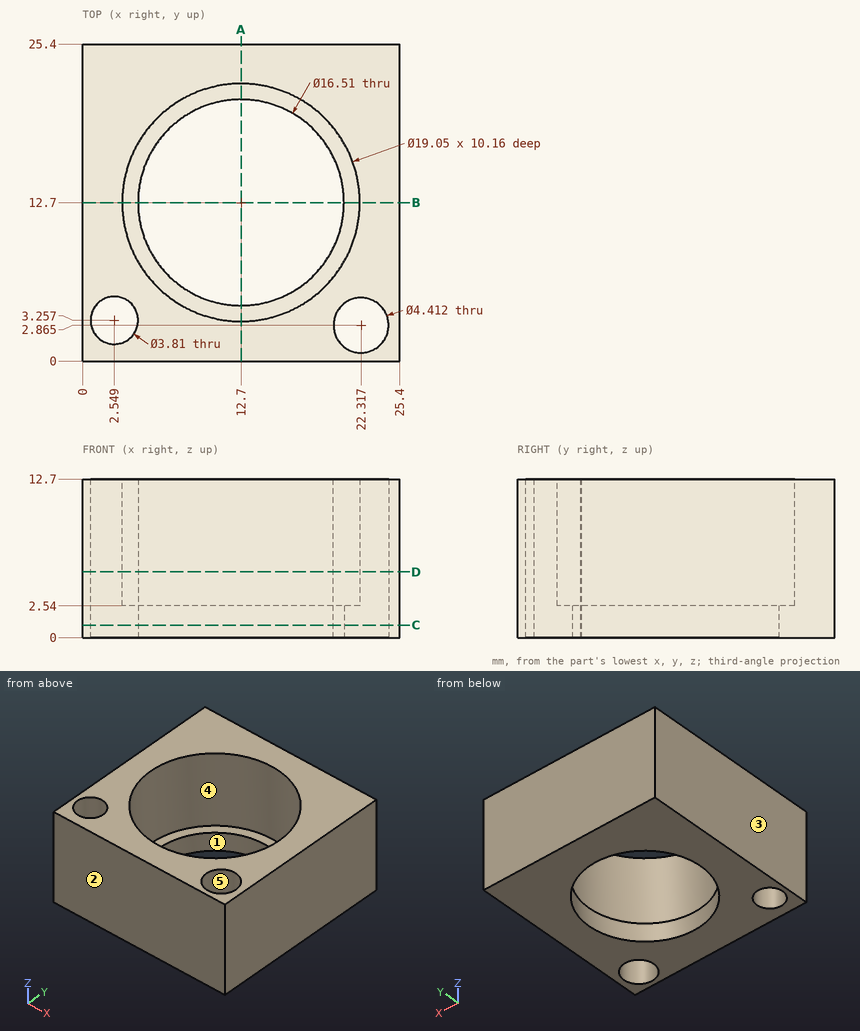
Here's the drawing with two shaded views (mm, measured from the low corner). I have some questions. A direction names the side the tool comes from. Give positions to 0.01 mm unless a question says otherwise; leave off trailing zeros. Order: outer loops, then holes, each group sorted by start corner. A loop starts at its lowest first (then second) coordinate and runs counter-clockwise, first axis right, second up. Notation, with made-up numbers: M 34,-3.5 L 89,-3.5 A5 cw 89,0.5 Z; hole C 2,37.5 d6. An arc over 180 degrees is marked long. Answer as a JSON object with one key per item and string values. Group by question number.
1) On a 3-axis mill with a long thin cutter (end or side, diameter ignored), from which of +Z, -Z, +X, -X, +Y, -Y can I reach the whole of each face in a straight line? I mean the marked faces 4 and 5. Say none if no direction works.
2) Suppose I cut it at C-C, the plane z = 1. Write out the boundary of the cut face in (x, y) (1 decimal).
3) Please list where these lines run through material, in increasing order: L1, parallel to Y at x = 12.7, z = 1.35 (1 decimal); L2, parallel to X at y = 3, z = 10.5 (1 decimal); L3, parallel to Y at x = 13, z = 9.5. Write a range as [from, to].
4) We'd pull the mould along X, two halves only. Please class the marked faces 1, 2 and 3: pulls with the +X half, pulls with the -X half, needs draft (parallel to the pull), parting line crosses it, or undercut.
5) Suppose I cut it at D-D, the plane z = 5.25. Count the separate pieces of the cut face and the enclosed holes in it.
6) Suppose I cut it at A-A, the plane x = 12.7. Write out the boundary of the cut face in (y, z) (1 decimal), plus the area to 3 significant figures.
Results found:
{
 "1": {"face 4": "+Z", "face 5": "+Z, -Z"},
 "2": {"outline": "M 0,0 L 25.4,0 L 25.4,25.4 L 0,25.4 Z; hole C 2.5,3.3 d3.8; hole C 12.7,12.7 d16.5; hole C 22.3,2.9 d4.4"},
 "3": {"L1": "[0, 4.4], [21, 25.4]", "L2": "[0, 0.7], [4.4, 20.1], [24.5, 25.4]", "L3": "[0, 3.18], [22.22, 25.4]"},
 "4": {"face 1": "undercut", "face 2": "needs draft", "face 3": "pulls with the -X half"},
 "5": {"separate pieces": "1", "enclosed holes": "3"},
 "6": {"outline": "M 0,0 L 4.4,0 L 4.4,2.5 L 3.2,2.5 L 3.2,12.7 L 0,12.7 Z; M 21,0 L 25.4,0 L 25.4,12.7 L 22.2,12.7 L 22.2,2.5 L 21,2.5 Z", "area": "87.1 mm²"}
}
